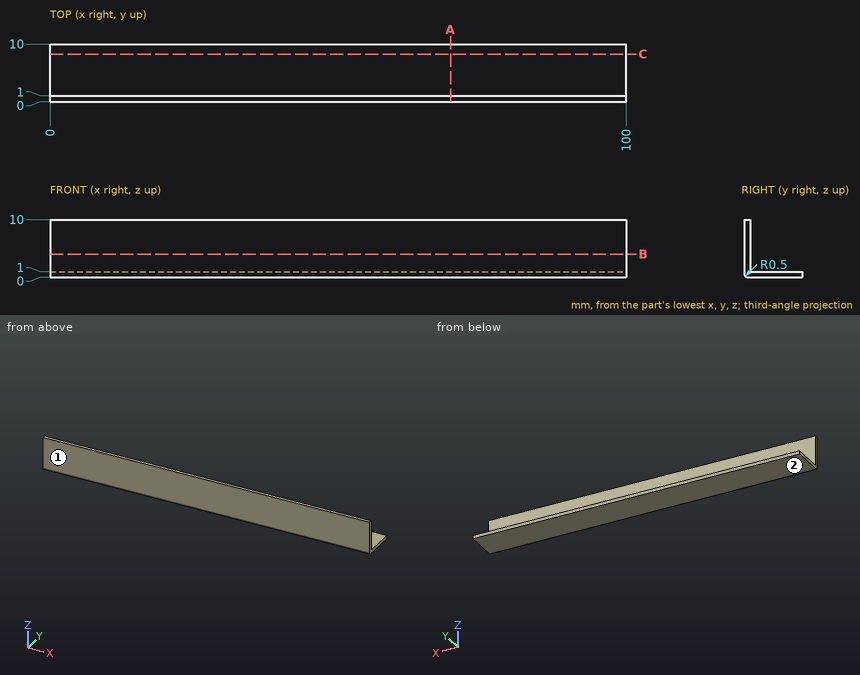
Geometry check sheet. Reference: drawing and pictorial views, mm from the part's lowest x, y, z. Give positions to 0.01 mm unless a question says otherwise; leave off trailing zeros. Order: outer loops, then holes, each group sorted by start corner. A loop starts at its lowest first (then second) coordinate and runs counter-clockwise, first axis right, second up. Notation, with made-up numbers: (86, 42.25) -> (138, 42.25) arc R33 ccw to (138, 73.25) -> close; hole circle Ø4 at (76, 11.5). An arc over 180 degrees is marked (long way). Use CSV: the item, a comma, the result in double quotes. Start each with the question number.
1) Material ranges on line 1 (Z direction, x = 58.5, y = 5.25), recorded low to high. Write a range as from..to.
2) Go/stop test with a flat-tipped pin: P1, Ø2.5, axis at x = 56, z = 5.5, coming from the +Y side. Record where the tip stops, or that it passes through.
3) Mould release check, pull along Z, two halves, no side actions. Record for the marked faces 1 and 2: released by +Z, released by -Z, zero draft, split by the parting line, or undercut.
4) Sectioned sample at B-B, the plane z = 4. Record the boundary of the cut face in (x, y).
5) Sectioned sample at A-A, the plane x = 69.5. Record the boundary of the cut face in (y, z).
Recorded:
1,line 1,"0..1"
2,P1,"y = 1"
3,face 1,"zero draft"
3,face 2,"released by -Z"
4,outline,"(0, 0) -> (100, 0) -> (100, 1) -> (0, 1) -> close"
5,outline,"(0, 0.5) arc R0.5 ccw to (0.5, 0) -> (10, 0) -> (10, 1) -> (1, 1) -> (1, 10) -> (0, 10) -> close"
